Job drawing, mm, ordinate dimensions from the low corner. One solid piece. A direction names the side the tool comes from. Give positions to 0.01 mm unless a question says otherwise; leave off trailing zeros. Write each loop counter-clockwise with the first axis right and the second up, starting at its lowest first coordinate (ties: lowest second). Pieces come first, ordered by that corner, then holes. Notation, with made-up numbers: M -3.5,57 L 49.5,57 A27 ccw 49.5,85 Z; hole C 89.25,-36.5 d2. An arc over 180 degrees is marked long. Answer as CSV lines item,"result". Start each with the question number.
Item 1: Band-saw the part on D-D, the plane y = 4.5. List the corners of the cut face in (x, z).
Item 2: Band-saw the part on A-A, the plane x = 15. List the corners of the cut face in (y, z).
Item 3: Band-saw the part on C-C, the plane y = 7. List the corners of the cut face in (x, z).
Item 4: Band-saw the part on B-B, the plane z = 15. List the corners of the cut face in (x, y).
Item 5: 3-axis set-ups, long thin cutter, end or side, ignore diameter. For the marked faces 1 and 2: which of +Z, -Z, +X, -X, +Y, -Y reach the whole face in a straight line?
Item 6: Pin check, flat tip, straight feed: pin 1 (1 mm diameter, centred on x = 17, y = 8, fed in from -Z). Stop position of the tip, or through.
Item 7: Wall check: L1, parallel to Y at x = 2, z = 15.25; L2, parallel to X at y = 8.5, z = 15; L3, parallel to Z at x = 10.25, y = 1. Give the ranges that are in metal, low to high. Write a range as from..to.
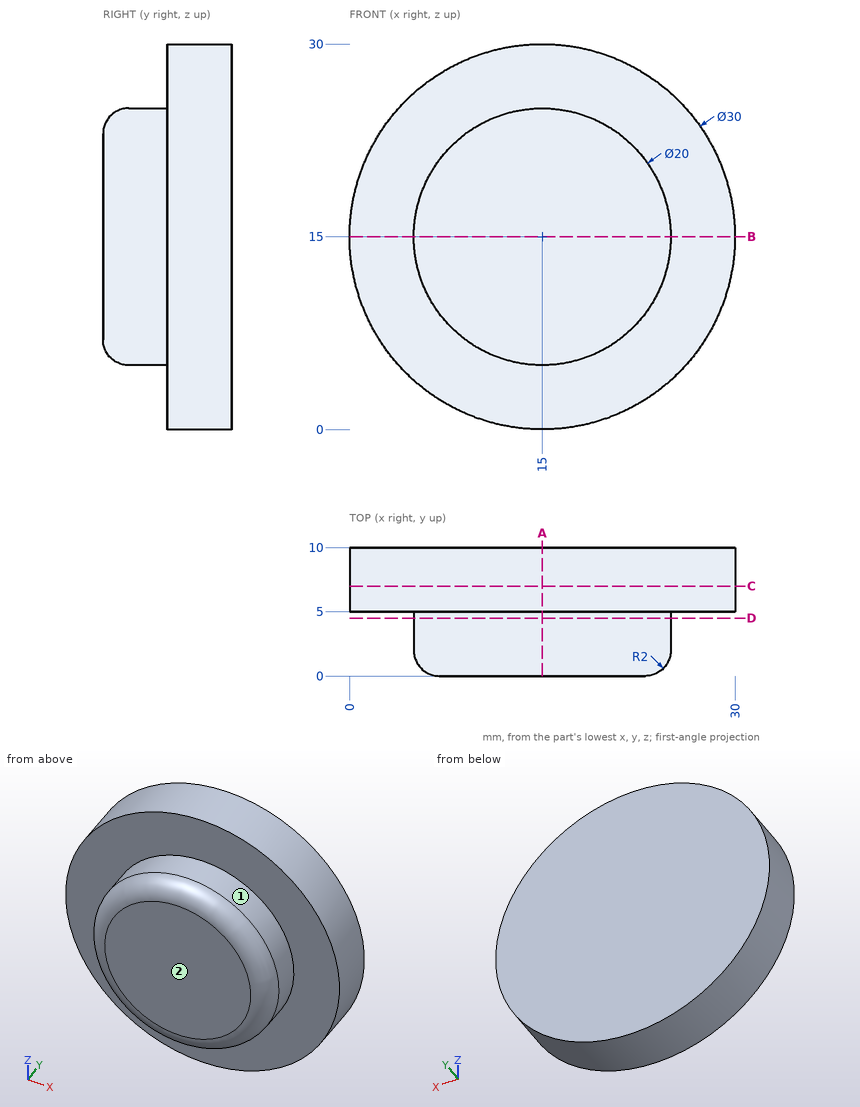
Output:
1,outline,"C 15,15 d20"
2,outline,"M 0,7 A2 ccw 2,5 L 5,5 L 5,0 L 10,0 L 10,30 L 5,30 L 5,25 L 2,25 A2 ccw 0,23 Z"
3,outline,"C 15,15 d30"
4,outline,"M 0,5 L 5,5 L 5,2 A2 ccw 7,0 L 23,0 A2 ccw 25,2 L 25,5 L 30,5 L 30,10 L 0,10 Z"
5,face 1,"-Y"
5,face 2,"+Z, -Z, +X, -X, -Y"
6,pin 1,"z = 0.08"
7,L1,"5..10"
7,L2,"0..30"
7,L3,"6.51..23.49"
